For this review, use the dimensioned drawing (mm, ordinates from the lowest corner) and the shaded views. Give positions to 0.01 mm unless a question says otherwise; leave off trailing zeros. Order: outer loops, then holes, each group sorted by start corner. A loop starts at its lowest first (then second) coordinate and runs counter-clockwise, first axis right, second up.
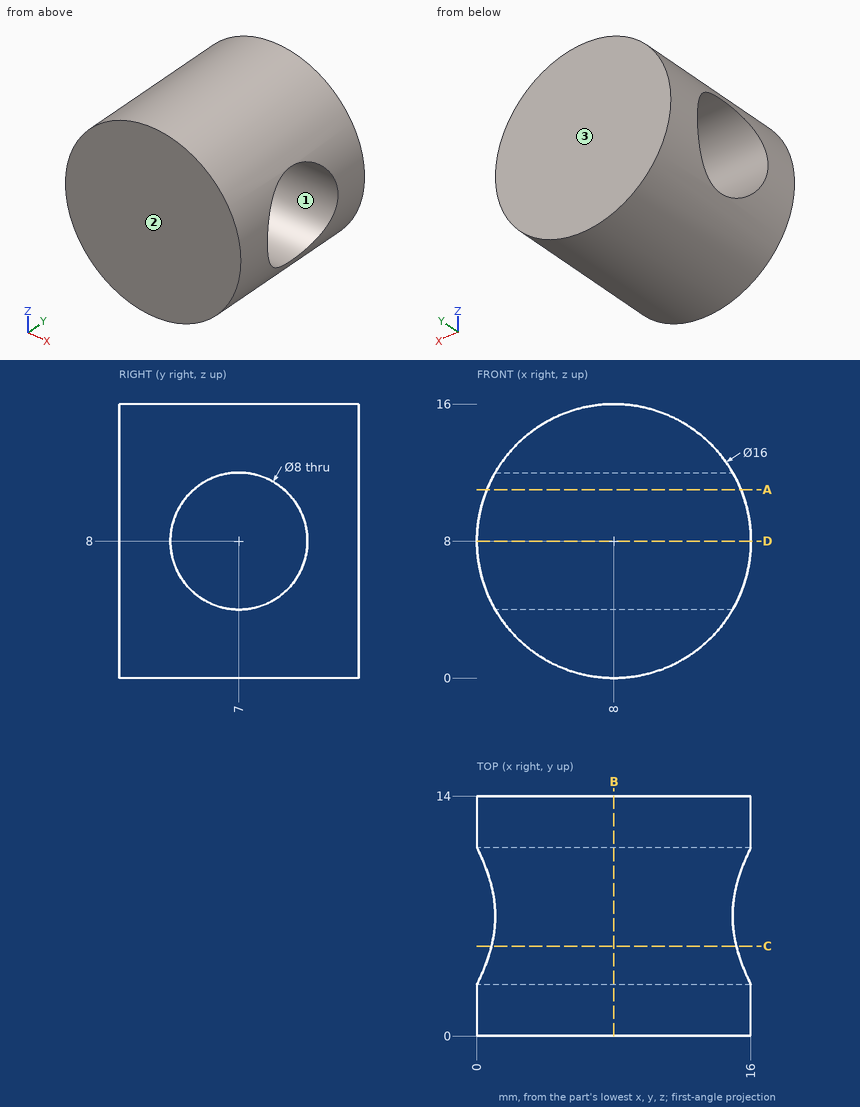
1. Take a section at D-D (z = 8). State the section outline as (x, y) points.
Recorded:
outline: (0, 0) - (16, 0) - (16, 3) - (0, 3) - close; (0, 11) - (16, 11) - (16, 14) - (0, 14) - close
2. For pin 1 (5 mm diameter, centred on y = 7, z = 8, fed in from +X); pin 2 (1 mm diameter, centred on x = 3, y = 6, fed in from +Z); pin 3 (5 mm diameter, centred on y = 6.5, z = 4.5, fed in from +X), all flat-tipped, find the tip position at first contact; note any pin that passes through.
Recorded:
pin 1: passes through
pin 2: stops at z = 14.61
pin 3: stops at x = 15.51
3. Take a section at C-C (y = 5.25). State the section outline as (x, z) points, then the cut area to 3 significant figures.
Recorded:
outline: (0.85, 4.4) arc R8 ccw to (15.15, 4.4) - close; (0.85, 11.6) - (15.15, 11.6) arc R8 ccw to start
area: 90.0 mm2
4. For line 1 along Y through (x, z) = (12.25, 8); line 2 along Y through (x, z) = (2.75, 5.75); line 3 along Z through (x, y) = (10.25, 6.25), list the stretches that pass through material, from the lowest coordinate up.
Recorded:
line 1: y = 0 to 3, 11 to 14
line 2: y = 0 to 3.69, 10.31 to 14
line 3: z = 0.32 to 4.07, 11.93 to 15.68
5. Take a section at B-B (x = 8). State the section outline as (y, z) points.
Recorded:
outline: (0, 0) - (14, 0) - (14, 16) - (0, 16) - close; hole circle Ø8 at (7, 8)
6. Take a section at A-A (z = 11). State the section outline as (x, y) points.
Recorded:
outline: (0.58, 0) - (15.42, 0) - (15.42, 4.35) - (0.58, 4.35) - close; (0.58, 9.65) - (15.42, 9.65) - (15.42, 14) - (0.58, 14) - close
7. Draft analysis for pull direction Y (two halves, no side actions). For the marked faces 1, 2 and 3, state which applies: pulls with the +Y half, pulls with the -Y half, needs draft (parallel to the pull), parting line crosses it, or undercut.
Recorded:
face 1: undercut
face 2: pulls with the -Y half
face 3: pulls with the +Y half
